Build history of the part. All positions in model axes, mm. A direction names the side the tool comes from. Coordinates: 2 decimals unless noted, no trailing zeros.
Item 1: Mould opens along X. For faces 3 (the face through (-25, 36, 0)), 4 (the face through (-22.5, 37, 19)), 5 (the face through (22.594, 37.389, 32.719)) say: released by +X, released by -X, zero draft, split by the parting line, or undercut.
Item 2: Flat gauge pin, fed straight in: pin 1 (2 mm diameter, centred on x = -2, z = 6.5, fed in from +Y). Where does the tip first touch, or does it go through?
Item 3: 3-axis set-ups, long thin cutter, end or side, ignore diameter. For faces 1 (the face through (22.719, 37.389, -32.594)), 2 (the face through (-21, 37.6, 32.5)): which of +Z, -Z, +X, -X, +Y, -Y reach the whole face in a straight line?
Item 4: Drill centre lines: line 1 along Y through (x, z) = (16.5, -4.5); line 2 along Y through (x, z) = (-16, -7.5); line 3 along Z through (x, y) = (22, 37.75) (3 decimals). Where is each one in solid material? Low to high.
from build123d import *

# Parameters (mm, degrees)
BOSS_EXTRUDE1_START = -35
BOSS_EXTRUDE1_DEPTH = 70
CUT_EXTRUDE1_DEPTH  = 61.466933282
FILLET1_R           = 8


# Read off the part's stored shape, not the designer's step: Boss-Extrude1
with BuildPart() as part:
    # Boss-Extrude1 outline → Boss-Extrude1 (new body)
    with BuildSketch(Plane.XY.offset(BOSS_EXTRUDE1_START)):
        with BuildLine():
            Line((25, 34.641016151), (25, 37.382028889))
            add(Edge.make_bspline(
                [(25, 37.382028889), (23.499149868, 38.038900322), (20.42020332, 39.233525172), (12.247727699, 41.641473317), (0, 43.149082804), (-12.247727699, 41.641473317), (-20.42020332, 39.233525172), (-23.499149868, 38.038900322), (-25, 37.382028889)],
                knots=[1.070195568, 1.070195568, 1.070195568, 1.070195568, 1.168370339, 1.266545109, 1.570796327, 1.875047544, 1.973222315, 2.071397085, 2.071397085, 2.071397085, 2.071397085], degree=3))
            Line((-25, 37.382028889), (-25, 34.641016151))
            add(Edge.make_bspline(
                [(25, 34.641016151), (0, 46.188021535), (-25, 34.641016151)],
                knots=[1.047197551, 1.047197551, 1.047197551, 2.094395102, 2.094395102, 2.094395102], degree=2, weights=[1, 0.866025404, 1]))
        make_face()
    extrude(amount=BOSS_EXTRUDE1_DEPTH)

    # Sketch5 → Cut-Extrude1 (cut, through all)
    with BuildSketch(Plane(origin=(0, 0, 0), x_dir=(1, 0, 0), z_dir=(0, 1, 0))):
        with BuildLine():
            Line((-22.5, -31), (-22.5, -6))
            ThreePointArc((-22.5, -6), (-21, -4.5), (-19.5, -6))
            Line((-19.5, -6), (-19.5, -31))
            ThreePointArc((-19.5, -31), (-21, -32.5), (-22.5, -31))
        make_face()
    extrude(amount=CUT_EXTRUDE1_DEPTH, mode=Mode.SUBTRACT)

    # Fillet1
    # the kernel refuses this fillet: 8 mm, written as the material it takes off along each edge
    with BuildSketch(Plane(origin=(-25, 57.382028889, -35), x_dir=(0, 0, 1), z_dir=(0, -1, 0)), Plane(origin=(-25, 57.382028889, 35), x_dir=(1, 0, 0), z_dir=(0, -1, 0)), Plane(origin=(25, 14.641016151, -35), x_dir=(0, 0, 1), z_dir=(0, 1, 0))) as fillet1_piece_1:
        with BuildLine():
            CenterArc((FILLET1_R, -FILLET1_R), FILLET1_R, 90, 90)
            Line((0, -FILLET1_R), (0, 0))
            Line((0, 0), (FILLET1_R, 0))
        make_face()
    extrude(amount=42.741012738, mode=Mode.SUBTRACT)
    with BuildSketch(Plane(origin=(25, 14.641016151, 35), x_dir=(0, 0, -1), z_dir=(0, 1, 0))) as fillet1_piece_2:
        with BuildLine():
            CenterArc((FILLET1_R, FILLET1_R), FILLET1_R, 180, 90)
            Line((0, FILLET1_R), (0, 0))
            Line((0, 0), (FILLET1_R, 0))
        make_face()
    extrude(amount=42.741012738, mode=Mode.SUBTRACT)


solid = part.part
Filled sheet:
1. face 3: released by -X
1. face 4: undercut
1. face 5: released by +X
2. pin 1: stops at y = 42.49
3. face 1: -Z, +X, +Y, -Y
3. face 2: +Y, -Y
4. line 1: y = 37.76 to 40.35
4. line 2: y = 37.9 to 40.48
4. line 3: z = -33.245 to 33.245
